Geometry check sheet. Reference: the model listing, model coordinates, mm. A direction names the side the tool comes from. Give positions to 0.01 mm unless a question says otherwise; leave off trailing zeros. Write each loop counter-clockwise with the first axis right and the second up, starting at its lowest first coordinate (ties: lowest second). Pieces come first, ordered by that corner, then holes. Notation, with made-up numbers: (59, -1) - (107, -1) arc R11 cw to (107, 20) - close; hole circle Ø6 at (44, -31.75). An arc over 180 degrees is marked (long way). Use a Markdown table: item, result.
Autodesk Inventor part; units mm, degrees
ref_plane "YZ Plane" through (0, 0, 0) normal (1, 0, 0) x (0, 1, 0)
ref_plane "XZ Plane" through (0, 0, 0) normal (0, 1, 0) x (-1, 0, 0)
ref_plane "XY Plane" through (0, 0, 0) normal (0, 0, 1) x (1, 0, 0)
sketch "Эскиз1" plane through (0, 0, 0) normal (0, 0, 1) x (1, 0, 0)
  line L0 (-13.1, -7) -> (13.1, -7) construction
  line L1 (13.1, -7) -> (13.1, 7) construction
  line L2 (13.1, 7) -> (-13.1, 7) construction
  line L3 (-13.1, 7) -> (-13.1, -7) construction
  line L4 (-13.1, -7) -> (13.1, 7) construction
  line L5 (13.1, -7) -> (-13.1, 7) construction
  line L6 (13.1, 7) -> (23.1, 7) construction
  line L7 (13.1, 5.35) -> (23.1, 5.35)
  line L8 (23.1, 8.65) -> (13.1, 8.65)
  arc A0 (13.1, 8.65) -> (13.1, 5.35) centre (13.1, 7) ccw
  arc A1 (23.1, 5.35) -> (23.1, 8.65) centre (23.1, 7) ccw
  line L9 (-26.1, -11.65) -> (26.1, -11.65)
  line L10 (26.1, -11.65) -> (26.1, 11.65)
  line L11 (26.1, 11.65) -> (-26.1, 11.65)
  line L12 (-26.1, 11.65) -> (-26.1, -11.65)
  line L13 (-26.1, -11.65) -> (26.1, 11.65) construction
  line L14 (26.1, -11.65) -> (-26.1, 11.65) construction
  line L15 (0, 0) -> (0, -11.65)
  line L16 (0, 0) -> (26.1, 0)
  line L17 (13.1, -5.35) -> (23.1, -5.35)
  line L18 (23.1, -8.65) -> (13.1, -8.65)
  arc A2 (13.1, -5.35) -> (13.1, -8.65) centre (13.1, -7) ccw
  arc A3 (23.1, -8.65) -> (23.1, -5.35) centre (23.1, -7) ccw
  line L19 (-13.1, 7) -> (-23.1, 7) construction
  line L20 (-13.1, 5.35) -> (-23.1, 5.35)
  line L21 (-23.1, 8.65) -> (-13.1, 8.65)
  arc A4 (-13.1, 5.35) -> (-13.1, 8.65) centre (-13.1, 7) ccw
  arc A5 (-23.1, 8.65) -> (-23.1, 5.35) centre (-23.1, 7) ccw
  line L22 (-13.1, -5.35) -> (-23.1, -5.35)
  arc A6 (-13.1, -8.65) -> (-13.1, -5.35) centre (-13.1, -7) ccw
  line L23 (-23.1, -8.65) -> (-13.1, -8.65)
  arc A7 (-23.1, -5.35) -> (-23.1, -8.65) centre (-23.1, -7) ccw
  point P0 (18.1, 7)
  point P1 (-18.1, 7)
  dimension "d0" = 14
  dimension "d1" = 26.2
  dimension "d2" = 10
  dimension "d3" = 3.3
  dimension "d4" = 3
  dimension "d5" = 3
extrude "Выдавливание1" add sketch "Эскиз1" along normal blind 4
properties part number "стена_каретка"
1) Section check A-A on y = -7. Record the boundary of the cut face in (x, z).
Working result:
| item | result |
|---|---|
| outline | (-26.1, 0) - (-24.75, 0) - (-24.75, 4) - (-26.1, 4) - close; (-11.45, 0) - (11.45, 0) - (11.45, 4) - (-11.45, 4) - close; (24.75, 0) - (26.1, 0) - (26.1, 4) - (24.75, 4) - close |
2) Set-up check for faces 1 (the flat face through (0, 0, 0)), 2 (the cylindrical face through (24.75, -6.96, 1.97)): record each of +Z, -Z, +X, -X, +Y, -Y from which the full face is reachable in a straight line by a thin tool's end or side.
Working result:
| item | result |
|---|---|
| face 1 | -Z, +X, -X, +Y, -Y |
| face 2 | +Z, -Z |
3) Section check B-B on x = -17. Record the boundary of the cut face in (y, z), then the cut area to 3 significant figures.
Working result:
| item | result |
|---|---|
| outline | (-11.65, 0) - (-8.65, 0) - (-8.65, 4) - (-11.65, 4) - close; (-5.35, 0) - (5.35, 0) - (5.35, 4) - (-5.35, 4) - close; (8.65, 0) - (11.65, 0) - (11.65, 4) - (8.65, 4) - close |
| area | 66.8 mm² |
4) Mould release check, pull along Y, two halves, no side actions. Record for faces 3 (the flat face through (0, 11.65, 2)), 4 (the flat face through (18, -8.65, 2)), 5 (the flat face through (18, -5.35, 2)), 6 (the flat face through (0, 0, 4)): pulls with the +Y half, pulls with the -Y half, needs draft (parallel to the pull), parting line crosses it, or undercut.
Working result:
| item | result |
|---|---|
| face 3 | pulls with the +Y half |
| face 4 | undercut |
| face 5 | undercut |
| face 6 | needs draft |
5) Section check C-C on z = 0.9. Record the boundary of the cut face in (x, y), then the cut area to 3 significant figures.
Working result:
| item | result |
|---|---|
| outline | (-26.1, -11.65) - (26.1, -11.65) - (26.1, 11.65) - (-26.1, 11.65) - close; hole (-23.1, -8.65) - (-13.1, -8.65) arc R1.65 ccw to (-13.1, -5.35) - (-23.1, -5.35) arc R1.65 ccw to start; hole (-23.1, 5.35) - (-13.1, 5.35) arc R1.65 ccw to (-13.1, 8.65) - (-23.1, 8.65) arc R1.65 ccw to start; hole (13.1, -8.65) - (23.1, -8.65) arc R1.65 ccw to (23.1, -5.35) - (13.1, -5.35) arc R1.65 ccw to start; hole (13.1, 5.35) - (23.1, 5.35) arc R1.65 ccw to (23.1, 8.65) - (13.1, 8.65) arc R1.65 ccw to start |
| area | 1,050 mm² |
6) Depth check by flat-ended pin: P1, Ø1.5, axis at x = -14, y = 3.5, coming from the -Z side. Enter the tip coordinate at first touch or a pass-through.
Working result:
| item | result |
|---|---|
| P1 | stops at z = 0 |
7) Material ranges on L1, parallel to Y at x = 13, z = 2.7; L2, parallel to X at y = 6.25, z = 3.05; L3, parallel to X at y = -8.5, z = 3.6, recorded low to high. Write a range as from..to.
Working result:
| item | result |
|---|---|
| L1 | y = -11.65..-8.65, -5.35..5.35, 8.65..11.65 |
| L2 | x = -26.1..-24.57, -11.63..11.63, 24.57..26.1 |
| L3 | x = -26.1..-23.79, -12.41..12.41, 23.79..26.1 |
